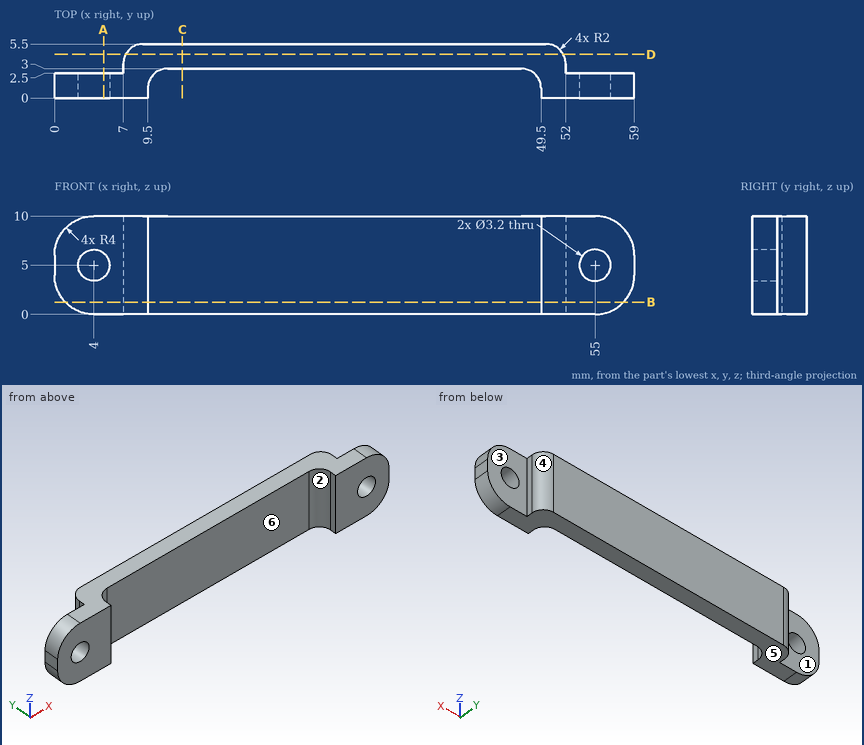
The figure shows three views and two pictorial views of one solid part (mm, origin at its lowest corner). Answer the questions. A direction names the side the tool comes from. Give positions to 0.01 mm unless a question says otherwise; leave off trailing zeros. Write each loop counter-clockwise with the first axis right and the second up, starting at its lowest first coordinate (ties: lowest second). Pieces come first, ordered by that corner, then holes. Notation, with made-up numbers: (-24.75, 68.5) -> (34.25, 68.5) arc R14 cw to (34.25, 90.5) -> close; hole circle Ø4 at (15.5, 1.5). An arc over 180 degrees is marked (long way). Use one line per item in the form item = value.
1) Each of these flat-tipped pins is pushed along its axis until it touches: P1, Ø4, axis at x = 4, z = 5, coming from the +Y side; P2, Ø4, axis at x = 49, z = 5, coming from the -Y side; P3, Ø3, axis at x = 36.5, z = 2.5, coming from the -Y side; P4, Ø2.5, axis at x = 55, z = 5, coming from the -Y side. Where does it stop, or does it pass through?
Result:
P1 = 2.5
P2 = 0
P3 = 3
P4 = through
2) Straight lines are drawn through the part: probe 1 along X at (y, z) = (0.65, 5); probe 2 along X at (y, z) = (1.5, 5); probe 3 along Z at (x, y) = (55, 1.55). For each, find the intervals that lie inside material, in ascending order.
Result:
probe_1 = 0 to 2.4, 5.6 to 9.5, 49.5 to 53.4, 56.6 to 59
probe_2 = 0 to 2.4, 5.6 to 9.56, 49.44 to 53.4, 56.6 to 59
probe_3 = 0 to 3.4, 6.6 to 10
3) Section D-D on y = 4.45 is taken. Write down the section's boundary in (x, z), plus the area to 3 significant figures.
Result:
outline = (7.24, 0) -> (51.76, 0) -> (51.76, 10) -> (7.24, 10) -> close
area = 445 mm²
4) Section C-C on x = 13 is taken. Write down the section's boundary in (y, z).
Result:
outline = (3, 0) -> (5.5, 0) -> (5.5, 10) -> (3, 10) -> close
5) Section B-B on z = 1.25 is taken. Write down the section's boundary in (x, y), plus the area to 3 significant figures.
Result:
outline = (1.1, 0) -> (9.5, 0) -> (9.5, 1) arc R2 cw to (11.5, 3) -> (47.5, 3) arc R2 cw to (49.5, 1) -> (49.5, 0) -> (57.9, 0) -> (57.9, 2.5) -> (52, 2.5) -> (52, 3.5) arc R2 ccw to (50, 5.5) -> (9, 5.5) arc R2 ccw to (7, 3.5) -> (7, 2.5) -> (1.1, 2.5) -> close
area = 157 mm²
6) For a pull along X with two mould halves and no side action, classify the marked faces 4, 5 and 6 as +X half, -X half, draft (parallel to the pull), parting line (faces both ways), or undercut.
Result:
face_4 = +X half
face_5 = draft
face_6 = undercut
7) Section A-A on x = 5 is taken. Write down the section's boundary in (y, z).
Result:
outline = (0, 0) -> (2.5, 0) -> (2.5, 3.75) -> (0, 3.75) -> close; (0, 6.25) -> (2.5, 6.25) -> (2.5, 10) -> (0, 10) -> close
8) A tool of negligible diameter and unlimited length cuts with its end or side. For the marked faces 1, 2 and 3, from which of +Z, -Z, +X, -X, +Y, -Y can it reach the whole face along a straight path? Write none if from no direction.
Result:
face_1 = +Z, -Z, -X, +Y
face_2 = +Z, -Z, -Y
face_3 = +Z, -Z, +X, +Y
